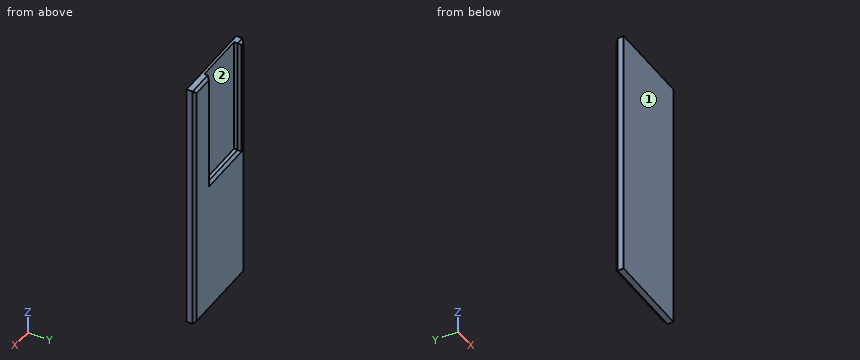
from build123d import *

# Parameters (mm, degrees)
SKETCH1_W           = 100
SKETCH1_H           = 300
BOSS_EXTRUDE1_DEPTH = 10
SKETCH2_W           = 60
SKETCH2_H           = 137.571747247
CUT_EXTRUDE1_DEPTH  = 7
CHAMFER1_SIZE       = 3


with BuildPart() as part:
    # Sketch1 → Boss-Extrude1 (new body)
    with BuildSketch(Plane(origin=(0, 0, 0), x_dir=(1, 0, 0), z_dir=(0, 1, 0))):
        Rectangle(SKETCH1_W, SKETCH1_H)
    extrude(amount=-BOSS_EXTRUDE1_DEPTH)

    # Sketch2 → Cut-Extrude1 (cut)
    with BuildSketch(Plane(origin=(0, 0, 0), x_dir=(1, 0, 0), z_dir=(0, 1, 0))):
        with Locations((-10.417468157, -81.214126377)):
            Rectangle(SKETCH2_W, SKETCH2_H)
    extrude(amount=-CUT_EXTRUDE1_DEPTH, mode=Mode.SUBTRACT)

    # Chamfer1
    chamfer1_edges = [part.edges().sort_by_distance(p)[0] for p in [
        (34.791265922, 0, 150),
        (19.582531843, 0, 81.214126377),
        (-10.417468157, 0, 12.428252753),
        (-40.417468157, 0, 81.214126377),
        (0, 0, -150),
        (50, 0, 0),
        (-45.208734078, 0, 150),
        (-50, 0, 0),
    ]]
    chamfer(chamfer1_edges, length=CHAMFER1_SIZE)


solid = part.part
Can you work these out from the model? Positions are in its coordinate system, mm. Face numbers are marked on the shaded views. Give positions to 0.01 mm unless a question says otherwise; leave off trailing zeros. Order: outer loops, then holes, each group sorted by start corner. A loop starts at its lowest first (then second) coordinate and runs counter-clockwise, first axis right, second up. Notation, with made-up numbers: M 10,45.25 L 26,45.25 A26 ccw 26,72.25 Z; hole C -24,-1 d1. An arc over 180 degrees is marked long. One line per item, written item: value.
Item 1: Please list where these lines run through material, in increasing order: line 1 (X direction, y = -6.25, z = 56); line 2 (Y direction, x = 7, z = 90); line 3 (Z direction, x = -30, y = -4).
Verdict:
line 1: -50 to -40.42, 19.58 to 50
line 2: -10 to -7
line 3: -150 to 12.43
Item 2: For pin 1 (1.2 mm diameter, centred on x = -4.5, y = -5, fed in from +Z), with a flat end and sliding along its axis, tell me the tip position at first contact or that it passes through.
Verdict:
pin 1: z = 12.43
Item 3: If we section it at B-B on x = -37.5: Write out the boundary of the cut face in (y, z), and give its area (3 significant figures).
Verdict:
outline: M -10,-150 L -3,-150 L 0,-147 L 0,9.43 L -3,12.43 L -7,12.43 L -7,150 L -10,150 Z
area: 2,030 mm2
Item 4: If we mould it in two halves opening along X, with no side actions, what happens to the marked faces 1 and 2? For each: pulls with the +X half, pulls with the -X half, needs draft (parallel to the pull), parting line crosses it, or undercut.
Verdict:
face 1: needs draft
face 2: undercut
Item 5: If we section it at A-A on z = 25: Write out the boundary of the cut face in (x, y).
Verdict:
outline: M -50,-10 L 50,-10 L 50,-3 L 47,0 L 22.58,0 L 19.58,-3 L 19.58,-7 L -40.42,-7 L -40.42,-3 L -43.42,0 L -47,0 L -50,-3 Z
